Build history of the part. All positions in model axes, mm. Face numbers are marked on the shaded views. A direction names the side the tool comes from. Round coordinates to 2 decimals unless told otherwise and drop trailing zeros. Write each loop counter-clockwise with the first axis right and the second up, starting at its lowest first coordinate (ties: lowest second). Pieces come first, ordered by that corner, then holes. Notation, with made-up numbers: M -10.75,58 L 2.25,58 A21 cw 2.25,95 Z; hole C 22.5,66 d4. An arc over 180 degrees is marked long. Use a Markdown table: item, result.
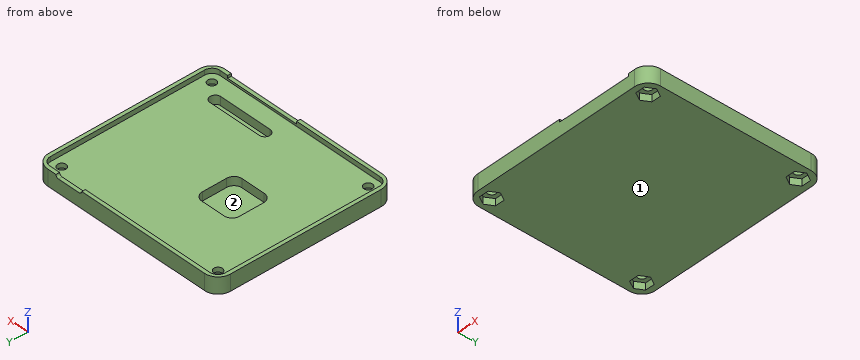
from build123d import *

# Parameters (mm, degrees)
SKETCH_1_W          = 73.73
SKETCH_1_H          = 66.24
EXTRUDE_1_DEPTH     = 6
CUT_EXTRUDE_1_DEPTH = 1.8
SKETCH_5_R          = 1.6
CUT_EXTRUDE_2_DEPTH = 100.204286702
CUT_EXTRUDE_3_DEPTH = 3.2
CUT_EXTRUDE_7_DEPTH = 9
SKETCH_11_W         = 28.050882838
SKETCH_11_H         = 1
CUT_EXTRUDE_8_DEPTH = 9
FILLET_1_R          = 5
CUT_EXTRUDE_9_DEPTH = 2.5


with BuildPart() as part:
    # 草图1 → 凸台-拉伸1 (new body)
    with BuildSketch(Plane.XY):
        with Locations((36.865, 33.12)):
            Rectangle(SKETCH_1_W, SKETCH_1_H)
    extrude(amount=EXTRUDE_1_DEPTH)

    # 草图2 → 切除-拉伸1 (cut)
    with BuildSketch(Plane.XY.offset(6)):
        with BuildLine():
            Line((4.36, 1.36), (69.37, 1.36))
            ThreePointArc((69.37, 1.36), (71.491320344, 2.238679656), (72.37, 4.36))
            Line((72.37, 4.36), (72.37, 61.88))
            ThreePointArc((72.37, 61.88), (71.491320344, 64.001320344), (69.37, 64.88))
            Line((69.37, 64.88), (4.36, 64.88))
            ThreePointArc((4.36, 64.88), (2.238679656, 64.001320344), (1.36, 61.88))
            Line((1.36, 61.88), (1.36, 4.36))
            ThreePointArc((1.36, 4.36), (2.238679656, 2.238679656), (4.36, 1.36))
        make_face()
    extrude(amount=-CUT_EXTRUDE_1_DEPTH, mode=Mode.SUBTRACT)

    # 草图5 → 切除-拉伸2 (cut, through all)
    with BuildSketch(Plane.XY.offset(4.2)):
        with Locations((5.115, 61.125)):
            Circle(SKETCH_5_R)
        with Locations(Location((68.615, 61.125, 0), (0, 0, 180))):
            Circle(SKETCH_5_R)
        with Locations((68.615, 5.115)):
            Circle(SKETCH_5_R)
        with Locations(Location((5.115, 5.115, 0), (0, 0, 180))):
            Circle(SKETCH_5_R)
    extrude(amount=-CUT_EXTRUDE_2_DEPTH, mode=Mode.SUBTRACT)

    # 草图6 → 切除-拉伸3 (cut)
    with BuildSketch(Plane.XY.offset(4.2)):
        with BuildLine():
            Line((62.307968064, 7.621116118), (42.256964224, 7.621116118))
            ThreePointArc((42.256964224, 7.621116118), (40.256964224, 9.621116118), (42.256964224, 11.621116118))
            Line((42.256964224, 11.621116118), (62.307968064, 11.621116118))
            ThreePointArc((62.307968064, 11.621116118), (64.307968064, 9.621116118), (62.307968064, 7.621116118))
        make_face()
        with BuildLine():
            Line((31.151031925, 43.266827275), (22.151031925, 43.266827275))
            ThreePointArc((22.151031925, 43.266827275), (20.029711582, 42.388147618), (19.151031925, 40.266827275))
            Line((19.151031925, 40.266827275), (19.151031925, 31.266827275))
            ThreePointArc((19.151031925, 31.266827275), (20.029711582, 29.145506931), (22.151031925, 28.266827275))
            Line((22.151031925, 28.266827275), (31.151031925, 28.266827275))
            ThreePointArc((31.151031925, 28.266827275), (33.272352269, 29.145506931), (34.151031925, 31.266827275))
            Line((34.151031925, 31.266827275), (34.151031925, 40.266827275))
            ThreePointArc((34.151031925, 40.266827275), (33.272352269, 42.388147618), (31.151031925, 43.266827275))
        make_face()
    extrude(amount=-CUT_EXTRUDE_3_DEPTH, mode=Mode.SUBTRACT)

    # 草图10 → 切除-拉伸7 (cut)
    with BuildSketch(Plane(origin=(0, 66.24, 0), x_dir=(1, 0, 0), z_dir=(0, 1, 0))):
        with BuildLine():
            Line((55.921832213, -5), (64.401832207, -5))
            ThreePointArc((64.401832207, -5), (65.108938988, -5.292893219), (65.401832207, -6))
            Line((65.401832207, -6), (54.921832213, -6))
            ThreePointArc((54.921832213, -6), (55.214725431, -5.292893219), (55.921832213, -5))
        make_face()
    extrude(amount=-CUT_EXTRUDE_7_DEPTH, mode=Mode.SUBTRACT)

    # 草图11 → 切除-拉伸8 (cut)
    with BuildSketch(Plane.XZ):
        with Locations((52.282673484, 5.5)):
            Rectangle(SKETCH_11_W, SKETCH_11_H)
    extrude(amount=-CUT_EXTRUDE_8_DEPTH, mode=Mode.SUBTRACT)

    # 圆角1
    fillet_1_edges = [part.edges().sort_by_distance(p)[0] for p in [
        (0, 66.24, 3),
        (73.73, 66.24, 3),
        (73.73, 0, 3),
        (0, 0, 3),
    ]]
    fillet(fillet_1_edges, radius=FILLET_1_R)

    # 草图12 → 切除-拉伸9 (cut)
    with BuildSketch(Plane(origin=(0, 0, 0), x_dir=(-1, 0, 0), z_dir=(0, 0, -1))):
        Polygon((-65.150898385, 61.125), (-66.882949192, 64.125), (-70.347050808, 64.125), (-72.079101615, 61.125), (-70.347050808, 58.125), (-66.882949192, 58.125), align=None)
        Polygon((-65.150898385, 5.115), (-66.882949192, 8.115), (-70.347050808, 8.115), (-72.079101615, 5.115), (-70.347050808, 2.115), (-66.882949192, 2.115), align=None)
        Polygon((-1.650898385, 5.115), (-3.382949192, 8.115), (-6.847050808, 8.115), (-8.579101615, 5.115), (-6.847050808, 2.115), (-3.382949192, 2.115), align=None)
        Polygon((-1.650898385, 61.125), (-3.382949192, 64.125), (-6.847050808, 64.125), (-8.579101615, 61.125), (-6.847050808, 58.125), (-3.382949192, 58.125), align=None)
    extrude(amount=-CUT_EXTRUDE_9_DEPTH, mode=Mode.SUBTRACT)


solid = part.part
Q1. Cut at B-B on y = 38. Give the cut face in (x, z).
Response values:
| item | result |
|---|---|
| outline | M 0,0 L 73.73,0 L 73.73,6 L 72.37,6 L 72.37,4.2 L 34.15,4.2 L 34.15,1 L 19.15,1 L 19.15,4.2 L 1.36,4.2 L 1.36,6 L 0,6 Z |
Q2. Cut at C-C on y = 19.5. Give the cut face in (x, z), and give its area (3 significant figures).
Response values:
| item | result |
|---|---|
| outline | M 0,0 L 73.73,0 L 73.73,6 L 72.37,6 L 72.37,4.2 L 1.36,4.2 L 1.36,6 L 0,6 Z |
| area | 315 mm2 |
Q3. Drop flat-ended pins along their axis: P1, Ø1.2, axis at x = 4.5, z = 0.5, coming from the +Y side; P2, Ø4, axis at x = 5.115, y = 61.125, coming from the +Z side. Give the stop position or say it passes through.
Response values:
| item | result |
|---|---|
| P1 | stops at y = 66.24 |
| P2 | stops at z = 4.2 |
Q4. Cut at A-A on x = 26. Give the cut face in (y, z), and give its area (3 significant figures).
Response values:
| item | result |
|---|---|
| outline | M 0,0 L 66.24,0 L 66.24,6 L 64.88,6 L 64.88,4.2 L 43.27,4.2 L 43.27,1 L 28.27,1 L 28.27,4.2 L 1.36,4.2 L 1.36,6 L 0,6 Z |
| area | 235 mm2 |
Q5. Drill centre lines: L1, parallel to Y at x = 20, z = 5.45; L2, parallel to Y at x = 67.5, z = 2.95; L3, parallel to Y at x = 49, z = 3.85. Where is each one in solid material? Low to high.
Response values:
| item | result |
|---|---|
| L1 | y = 0 to 1.36, 64.88 to 66.24 |
| L2 | y = 0 to 3.97, 6.26 to 59.98, 62.27 to 66.24 |
| L3 | y = 0 to 7.62, 11.62 to 66.24 |
Q6. Which spindle directions (+Z, -Z, +X, -X, +Y, -Y) get a long thin tool onto all of the face, cutting with end or side? Do the marked faces 1 and 2. Say none if no direction does.
Response values:
| item | result |
|---|---|
| face 1 | -Z, +X, -X, +Y, -Y |
| face 2 | +Z |
